Verification items for the finished model (mm, model axes). Face numbers are marked on the shaded views. A direction names the side the tool comes from. Round coordinates to 2 decimals unless told otherwise and drop trailing zeros. Write each loop counter-clockwise with the first axis right and the second up, starting at its lowest first coordinate (ties: lowest second). Pieces come first, ordered by that corner, then holes. Notation, with made-up numbers: M 63,64.5 L 76,64.5 A22 cw 76,95.5 Z; hole C -28,-40 d4. An arc over 180 degrees is marked long. Answer in a Markdown table with one row per item. Add a question column.
1. Go/stop test with flat-tipped pins: pin 1 Ø4 at (y, z) = (14, 2.5) entering from +X; pin 2 Ø4 at (x, z) = (4, 10) entering from +Y; pin 3 Ø4 at (x, z) = (10.5, 6.5) entering from +Y. Record where each tip stops, or that it passes through.
2. Sectioned sample at D-D on y = 16. Record the cut outline in (x, z), plus the area to 3 significant figures.
3. Set-up check for the marked faces 5 and 6: record each of +Z, -Z, +X, -X, +Y, -Y from which the full face is reachable in a straight line by a thin tool's end or side.
4. Sectioned sample at C-C on x = 0. Record the cut outline in (y, z).
5. Material ranges on probe 1 along X at (y, z) = (1.2, 0); probe 2 along Y at (x, z) = (-3, 11.75); probe 3 along X at (y, z) = (13.5, -1), recorded low to high.
6. Draft check along Y on the marked faces 1, 2, 3 and 4. Enter one of: pulls with the +Y half, pulls with the -Y half, needs draft (parallel to the pull), parting line crosses it, or undercut.
7. Sectioned sample at B-B on z = 0. Record the cut outline in (x, y).
8. Sectioned sample at A-A on y = 3. Record the cut outline in (x, z) (1 decimal), plus the area to 3 significant figures.
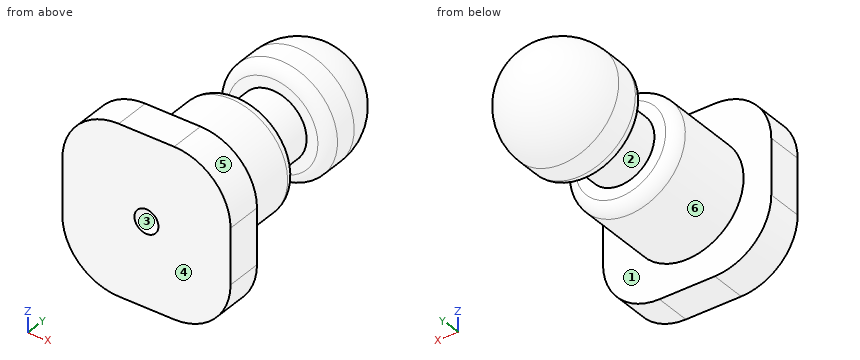
```python
from build123d import *

# Parameters (mm, degrees)
SKETCH2_W               = 29.8
SKETCH2_H               = 29.8
BOSS_EXTRUDE1_DEPTH     = 6.35
FILLET1_R               = 10
SKETCH9_R               = 10
BOSS_EXTRUDE6_DEPTH     = 40
FILLET5_R               = 10
CUT_EXTRUDE2_DEPTH      = 4
CUT_EXTRUDE2_DEPTH_BACK = 4
SKETCH11_R              = 10
SKETCH11_R_2            = 6
FILLET6_R               = 2
SKETCH12_R              = 2.1225
CUT_EXTRUDE3_DEPTH      = 5


with BuildPart() as part:
    # Sketch2 → Boss-Extrude1 (new body)
    with BuildSketch(Plane(origin=(0, 0, 0), x_dir=(1, 0, 0), z_dir=(0, 1, 0))):
        Rectangle(SKETCH2_W, SKETCH2_H)
    extrude(amount=BOSS_EXTRUDE1_DEPTH)

    # Fillet1
    fillet1_edges = [part.edges().sort_by_distance(p)[0] for p in [
        (-14.9, 3.175, -14.9),
        (14.9, 3.175, -14.9),
        (14.9, 3.175, 14.9),
        (-14.9, 3.175, 14.9),
    ]]
    fillet(fillet1_edges, radius=FILLET1_R)

    # Sketch9 → Boss-Extrude6 (add)
    with BuildSketch(Plane(origin=(0, 6.35, 0), x_dir=(1, 0, 0), z_dir=(0, 1, 0))):
        with Locations(Location((0, 0, 0), (0, 0, 270))):
            Circle(SKETCH9_R)
    extrude(amount=BOSS_EXTRUDE6_DEPTH)

    # Fillet5
    fillet5_edges = [part.edges().sort_by_distance(p)[0] for p in [
        (0, 46.35, -10),
    ]]
    fillet(fillet5_edges, radius=FILLET5_R)

    # Sketch11 → Cut-Extrude2 (cut, two sides: drawn at the far end of the back side and taken through both)
    with BuildSketch(Plane(origin=(0, 26.35, 0), x_dir=(1, 0, 0), z_dir=(0, 1, 0)).offset(-CUT_EXTRUDE2_DEPTH_BACK)):
        with Locations(Location((0, 0, 0), (0, 0, 270))):
            Circle(SKETCH11_R)
        with Locations(Location((0, 0, 0), (0, 0, 270))):
            Circle(SKETCH11_R_2, mode=Mode.SUBTRACT)
    extrude(amount=CUT_EXTRUDE2_DEPTH + CUT_EXTRUDE2_DEPTH_BACK, mode=Mode.SUBTRACT)

    # Fillet6
    fillet6_edges = [part.edges().sort_by_distance(p)[0] for p in [
        (0, 30.35, -10),
        (0, 22.35, -10),
    ]]
    fillet(fillet6_edges, radius=FILLET6_R)

    # Sketch12 → Cut-Extrude3 (cut)
    with BuildSketch(Plane.XZ):
        with Locations(Location((0, 0, 0), (0, 0, 270))):
            Circle(SKETCH12_R)
    extrude(amount=-CUT_EXTRUDE3_DEPTH, mode=Mode.SUBTRACT)


solid = part.part
```
Geometry check:
| question | item | result |
|---|---|---|
| 1 | pin 1 | stops at x = 9.99 |
| 1 | pin 2 | stops at y = 41.15 |
| 1 | pin 3 | stops at y = 6.35 |
| 2 | outline | C 0,0 d20 |
| 2 | area | 314 mm2 |
| 3 | face 5 | +Z, +X, +Y, -Y |
| 3 | face 6 | +Y |
| 4 | outline | M 0,-14.9 L 6.35,-14.9 L 6.35,-10 L 20.35,-10 A2 ccw 22.35,-8 L 22.35,-6 L 30.35,-6 L 30.35,-8 A2 ccw 32.35,-10 L 36.35,-10 A10 ccw 36.35,10 L 32.35,10 A2 ccw 30.35,8 L 30.35,6 L 22.35,6 L 22.35,8 A2 ccw 20.35,10 L 6.35,10 L 6.35,14.9 L 0,14.9 L 0,2.12 L 5,2.12 L 5,-2.12 L 0,-2.12 Z |
| 5 | probe 1 | x = -14.9 to -2.12, 2.12 to 14.9 |
| 5 | probe 2 | y = 0 to 6.35 |
| 5 | probe 3 | x = -9.95 to 9.95 |
| 6 | face 1 | pulls with the +Y half |
| 6 | face 2 | undercut |
| 6 | face 3 | needs draft |
| 6 | face 4 | pulls with the -Y half |
| 7 | outline | M -14.9,0 L -2.12,0 L -2.12,5 L 2.12,5 L 2.12,0 L 14.9,0 L 14.9,6.35 L 10,6.35 L 10,20.35 A2 ccw 8,22.35 L 6,22.35 L 6,30.35 L 8,30.35 A2 ccw 10,32.35 L 10,36.35 A10 ccw -10,36.35 L -10,32.35 A2 ccw -8,30.35 L -6,30.35 L -6,22.35 L -8,22.35 A2 ccw -10,20.35 L -10,6.35 L -14.9,6.35 Z |
| 8 | outline | M -14.9,-4.9 A10 ccw -4.9,-14.9 L 4.9,-14.9 A10 ccw 14.9,-4.9 L 14.9,4.9 A10 ccw 4.9,14.9 L -4.9,14.9 A10 ccw -14.9,4.9 Z; hole C 0,0 d4.2 |
| 8 | area | 788 mm2 |
